```python
from build123d import *

# Parameters (mm, degrees)
SKETCH11_R          = 73.025
SKETCH11_R_2        = 42.926
SKETCH11_R_3        = 5.588
BOSS_EXTRUDE3_DEPTH = 7.874
SKETCH12_R          = 73.025
SKETCH12_R_2        = 65.151
BOSS_EXTRUDE4_DEPTH = 30.226
BOSS_EXTRUDE5_START = -7.874
SKETCH19_R          = 5.588
BOSS_EXTRUDE5_DEPTH = 7.874


with BuildPart() as part:
    # Sketch11 → Boss-Extrude3 (new body)
    with BuildSketch(Plane(origin=(0, 0, 0), x_dir=(1, 0, 0), z_dir=(0, 1, 0))):
        with Locations(Location((0, 0, 0), (0, 0, 270))):
            Circle(SKETCH11_R)
        with Locations(Location((0, 0, 0), (0, 0, 270))):
            Circle(SKETCH11_R_2, mode=Mode.SUBTRACT)
        with Locations(Location((0, -54.102, 0), (0, 0, 270))):
            Circle(SKETCH11_R_3, mode=Mode.SUBTRACT)
        with Locations(Location((-38.255891076, -38.255891076, 0), (0, 0, 270))):
            Circle(SKETCH11_R_3, mode=Mode.SUBTRACT)
        with Locations(Location((-54.102, 0, 0), (0, 0, 270))):
            Circle(SKETCH11_R_3, mode=Mode.SUBTRACT)
        with Locations(Location((-38.255891076, 38.255891076, 0), (0, 0, 270))):
            Circle(SKETCH11_R_3, mode=Mode.SUBTRACT)
        with Locations(Location((0, 54.102, 0), (0, 0, 270))):
            Circle(SKETCH11_R_3, mode=Mode.SUBTRACT)
        with Locations(Location((38.255891076, 38.255891076, 0), (0, 0, 270))):
            Circle(SKETCH11_R_3, mode=Mode.SUBTRACT)
        with Locations(Location((54.102, 0, 0), (0, 0, 270))):
            Circle(SKETCH11_R_3, mode=Mode.SUBTRACT)
        with Locations(Location((38.255891076, -38.255891076, 0), (0, 0, 270))):
            Circle(SKETCH11_R_3, mode=Mode.SUBTRACT)
    extrude(amount=BOSS_EXTRUDE3_DEPTH)

    # Sketch12 → Boss-Extrude4 (add)
    with BuildSketch(Plane(origin=(0, 7.874, 0), x_dir=(1, 0, 0), z_dir=(0, 1, 0))):
        with Locations(Location((0, 0, 0), (0, 0, 270))):
            Circle(SKETCH12_R)
        with Locations(Location((0, 0, 0), (0, 0, 270))):
            Circle(SKETCH12_R_2, mode=Mode.SUBTRACT)
    extrude(amount=BOSS_EXTRUDE4_DEPTH)

    # Sketch19 → Boss-Extrude5 (add)
    # profile 1 of 4: a face of its own
    with BuildSketch(Plane(origin=(0, 38.1, 0), x_dir=(1, 0, 0), z_dir=(0, 1, 0)).offset(BOSS_EXTRUDE5_START)):
        with BuildLine():
            Line((-11.176, -54.102), (-11.176, -72.164725795))
            Line((-11.176, -72.164725795), (11.176, -72.164725795))
            Line((11.176, -72.164725795), (11.176, -54.102))
            ThreePointArc((11.176, -54.102), (0, -42.926), (-11.176, -54.102))
        make_face()
        with Locations(Location((0, -54.102, 0), (0, 0, 270))):
            Circle(SKETCH19_R, mode=Mode.SUBTRACT)
    # profile 2 of 4: a face of its own
    with BuildSketch(Plane(origin=(0, 38.1, 0), x_dir=(1, 0, 0), z_dir=(0, 1, 0)).offset(BOSS_EXTRUDE5_START)):
        with BuildLine():
            Line((-54.102, 11.176), (-72.164725795, 11.176))
            Line((-72.164725795, 11.176), (-72.164725795, -11.176))
            Line((-72.164725795, -11.176), (-54.102, -11.176))
            ThreePointArc((-54.102, -11.176), (-42.926, 0), (-54.102, 11.176))
        make_face()
        with Locations(Location((-54.102, 0, 0), (0, 0, 270))):
            Circle(SKETCH19_R, mode=Mode.SUBTRACT)
    # profile 3 of 4: a face of its own
    with BuildSketch(Plane(origin=(0, 38.1, 0), x_dir=(1, 0, 0), z_dir=(0, 1, 0)).offset(BOSS_EXTRUDE5_START)):
        with BuildLine():
            Line((11.176, 54.102), (11.176, 72.164725795))
            Line((11.176, 72.164725795), (-11.176, 72.164725795))
            Line((-11.176, 72.164725795), (-11.176, 54.102))
            ThreePointArc((-11.176, 54.102), (0, 42.926), (11.176, 54.102))
        make_face()
        with Locations(Location((0, 54.102, 0), (0, 0, 270))):
            Circle(SKETCH19_R, mode=Mode.SUBTRACT)
    # profile 4 of 4: a face of its own
    with BuildSketch(Plane(origin=(0, 38.1, 0), x_dir=(1, 0, 0), z_dir=(0, 1, 0)).offset(BOSS_EXTRUDE5_START)):
        with BuildLine():
            Line((54.102, -11.176), (72.164725795, -11.176))
            Line((72.164725795, -11.176), (72.164725795, 11.176))
            Line((72.164725795, 11.176), (54.102, 11.176))
            ThreePointArc((54.102, 11.176), (42.926, 0), (54.102, -11.176))
        make_face()
        with Locations(Location((54.102, 0, 0), (0, 0, 270))):
            Circle(SKETCH19_R, mode=Mode.SUBTRACT)
    extrude(amount=BOSS_EXTRUDE5_DEPTH)


solid = part.part
```
Verification items for the finished model (mm, model axes). A direction names the side the tool comes from. Coordinates: 2 decimals unless noted, no trailing zeros. Loops run counter-clockwise (first coordinate to the right, second up) from the corner with the lowest first, then second, coordinate; pieces in that order, holes last. Notation, with made-up numbers: (16, 20) - (59, 20) arc R31 ccw to (59, 59) - close; hole circle Ø10 at (13.25, -19.75). An arc over 180 degrees is marked (long way). Answer as a JSON object with one key per item and string values.
(1) Access from +Z, -Z, +X, -X, +Y, -Y to the whole of each face (thin tool, end or side, straight path). Record for faces 4 (the flat face through (-59, 34, -11.176)), 5 (the flat face through (-59, 30.226, -3)), 6 (the cylindrical face through (-2.14, 3.882, 59.264)).
Response:
{"face 4": "+Y", "face 5": "none", "face 6": "+Y, -Y"}
(2) Cross-section at A-A, the plane z = 0. Count the separate pieces of the cut face and the enclosed holes in it, then the cut area to 3 significant figures.
Response:
{"separate pieces": "6", "enclosed holes": "0", "area": "948 mm²"}
(3) Scan lines: line 1 along X through (y, z) = (16.5, -2); line 2 along Z through (x, y) = (-38, 4.5); line 3 along Z through (x, y) = (0, 17) (3 decimals). Record each from-to range of solid material in increasing order.
Response:
{"line 1": "x = -73 to -65.12, 65.12 to 73", "line 2": "z = -62.36 to -43.84, -32.67 to -19.97, 19.97 to 32.67, 43.84 to 62.36", "line 3": "z = -73.025 to -65.151, 65.151 to 73.025"}
(4) Mould release check, pull along Y, two halves, no side actions. Record for faces 1 (the flat face through (-31, 0, 31)), 2 (the flat face through (-3, 30.226, -59)), 3 (the flat face through (-11.176, 34, 59)): pulls with the +Y half, pulls with the -Y half, needs draft (parallel to the pull), parting line crosses it, or undercut.
Response:
{"face 1": "pulls with the -Y half", "face 2": "undercut", "face 3": "needs draft"}
(5) Cross-section at C-C, the plane z = -23. Record the boundary of the cut face in (x, y), then the cut area to 3 significant figures.
Response:
{"outline": "(-69.31, 0) - (-36.24, 0) - (-36.24, 7.87) - (-60.96, 7.87) - (-60.96, 38.1) - (-69.31, 38.1) - close; (36.24, 0) - (69.31, 0) - (69.31, 38.1) - (60.96, 38.1) - (60.96, 7.87) - (36.24, 7.87) - close", "area": "1,030 mm²"}
(6) Cross-section at D-D, the plane z = -57.5. Record the boundary of the cut face in (x, y), then the cut area to 3 significant figures.
Response:
{"outline": "(-45.02, 0) - (-4.44, 0) - (-4.44, 7.87) - (-30.63, 7.87) - (-30.63, 38.1) - (-45.02, 38.1) - close; (-11.18, 30.23) - (-4.44, 30.23) - (-4.44, 38.1) - (-11.18, 38.1) - close; (4.44, 0) - (45.02, 0) - (45.02, 38.1) - (30.63, 38.1) - (30.63, 7.87) - (4.44, 7.87) - close; (4.44, 30.23) - (11.18, 30.23) - (11.18, 38.1) - (4.44, 38.1) - close", "area": "1,610 mm²"}
(7) Go/stop test with flat-tipped pins: pin 1 Ø3 at (x, y) = (5, 27) entering from +Z; pin 2 Ø9 at (x, z) = (-38.26, 38.26) entering from -Y; pin 3 Ø1 at (x, z) = (-37.5, 51) entering from +Y; pin 4 Ø8 at (x, y) = (29.5, 8) entering from -Z. Record where each tip stops, or that it passes through.
Response:
{"pin 1": "stops at z = 72.94", "pin 2": "passes through", "pin 3": "stops at y = 7.87", "pin 4": "stops at z = -68.43"}
